Could you check a few things on this model? Use its own coordinates, in mm. Face numbers are marked on the shaded views. Give positions to 0.01 mm unless a question says otherwise; leave off trailing zeros. Order: outer loops, then holes, each group sorted by start corner. A loop starts at its lowest first (then second) coordinate and runs counter-clockwise, first axis right, second up. Notation, with made-up numbers: M 13,19.5 L 34,19.5 A31 ccw 34,43.5 Z; hole C 24,61 d6. An arc over 180 degrees is marked long. Use a Markdown table: item, result. Add a question column.
Item 1: Suppose I cut it at B-B on x = 10.5. Write out the boundary of the cut face in (y, z), plus the area to 3 significant figures.
Item 2: If I drill on L1, parallel to X at y = 14.75, z = -1; L2, parallel to Y at x = -20.5, z = 9; L3, parallel to Y at x = 17, z = 17, over which ranges is the centre line in solid material (lowest first)? Write a range as from..to.
Item 3: I'm going to push a flat-ended pin straight in: pin 1 Ø6 at (y, z) = (18, 7) entering from +X. Where does the tip first touch, or does it pass through?
Item 4: Suppose I cut it at C-C on x = 17. Write out the boundary of the cut face in (y, z), plus the area to 3 significant figures.
Item 5: Suppose I cut it at D-D on z = -5. Write out the boundary of the cut face in (x, y).
Item 6: If we mould it in two halves opening along Z, with no side actions, what happens to the marked faces 1, 2, 3 and 4? For each: released by +Z, released by -Z, zero draft, split by the parting line, or undercut.
Item 7: Suppose I cut it at A-A on y = 15. Write out the boundary of the cut face in (x, z), plus the area to 3 significant figures.
from build123d import *

# Parameters (mm, degrees)
SKETCH1_W               = 48
SKETCH1_H               = 45
BOSS_EXTRUDE1_DEPTH     = 30
SKETCH2_W               = 10.2
SKETCH2_H               = 20.2
CUT_EXTRUDE1_DEPTH      = 45
SKETCH3_R               = 4.15
CUT_EXTRUDE2_DEPTH      = 46
CUT_EXTRUDE3_DEPTH      = 1
CUT_EXTRUDE3_DEPTH_BACK = 31


with BuildPart() as part:
    # Sketch1 → Boss-Extrude1 (new body)
    with BuildSketch(Plane(origin=(0, 0, 0), x_dir=(1, 0, 0), z_dir=(0, 1, 0))):
        Rectangle(SKETCH1_W, SKETCH1_H)
    extrude(amount=BOSS_EXTRUDE1_DEPTH)

    # Sketch2 → Cut-Extrude1 (cut)
    with BuildSketch(Plane(origin=(24, 0, 0), x_dir=(0, 0, -1), z_dir=(1, 0, 0))):
        with Locations((-9, 15)):
            Rectangle(SKETCH2_W, SKETCH2_H)
    extrude(amount=-CUT_EXTRUDE1_DEPTH, mode=Mode.SUBTRACT)

    # Sketch3 → Cut-Extrude2 (cut, through all)
    with BuildSketch(Plane.XY.offset(22.5)):
        with Locations((-17, 15)):
            Circle(SKETCH3_R)
        with Locations((17, 15)):
            Circle(SKETCH3_R)
    extrude(amount=-CUT_EXTRUDE2_DEPTH, mode=Mode.SUBTRACT)

    # Sketch4 → Cut-Extrude3 (cut, two sides)
    with BuildSketch(Plane(origin=(0, 30, 0), x_dir=(1, 0, 0), z_dir=(0, 1, 0))) as cut_extrude3_sk:
        with BuildLine():
            Line((-7, 141.788608739), (-7, 22.5))
            ThreePointArc((-7, 22.5), (0, 15.5), (7, 22.5))
            Line((7, 22.5), (7, 141.788608739))
            Line((7, 141.788608739), (7, 380.365826216))
            Line((7, 380.365826216), (-7, 380.365826216))
            Line((-7, 380.365826216), (-7, 141.788608739))
        make_face()
    extrude(amount=CUT_EXTRUDE3_DEPTH, mode=Mode.SUBTRACT)
    extrude(cut_extrude3_sk.sketch, amount=-CUT_EXTRUDE3_DEPTH_BACK, mode=Mode.SUBTRACT)


solid = part.part
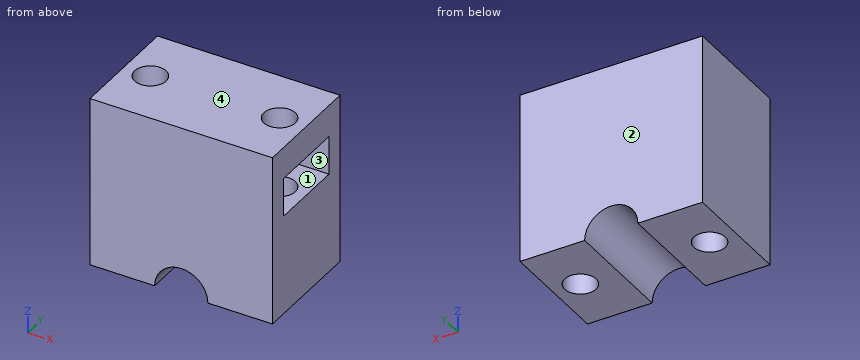
Findings below:
| question | item | result |
|---|---|---|
| 1 | outline | M 0,-22.5 L 30,-22.5 L 30,22.5 L 0,22.5 Z; hole M 4.9,3.9 L 25.1,3.9 L 25.1,14.1 L 4.9,14.1 Z |
| 1 | area | 1,140 mm^2 |
| 2 | L1 | x = -24..-21.14, -12.86..12.86, 21.14..24 |
| 2 | L2 | y = 0..4.9, 25.1..30 |
| 2 | L3 | y = 0..10.85, 19.15..30 |
| 3 | pin 1 | stops at x = -21 |
| 4 | outline | M 0,-22.5 L 10.85,-22.5 L 10.85,3.9 L 4.9,3.9 L 4.9,14.1 L 10.85,14.1 L 10.85,22.5 L 0,22.5 Z; M 19.15,-22.5 L 30,-22.5 L 30,22.5 L 19.15,22.5 L 19.15,14.1 L 25.1,14.1 L 25.1,3.9 L 19.15,3.9 Z |
| 4 | area | 855 mm^2 |
| 5 | outline | M -24,0 L 24,0 L 24,30 L -24,30 Z; hole C -17,15 d8.3; hole C 17,15 d8.3 |
| 6 | face 1 | undercut |
| 6 | face 2 | zero draft |
| 6 | face 3 | undercut |
| 6 | face 4 | released by +Z |
| 7 | outline | M -24,-22.5 L -21.15,-22.5 L -21.15,22.5 L -24,22.5 Z; M -12.85,-22.5 L -7,-22.5 A7 cw 7,-22.5 L 12.85,-22.5 L 12.85,3.9 L -12.85,3.9 Z; M -12.85,14.1 L 12.85,14.1 L 12.85,22.5 L -12.85,22.5 Z; M 21.15,-22.5 L 24,-22.5 L 24,3.9 L 21.15,3.9 Z; M 21.15,14.1 L 24,14.1 L 24,22.5 L 21.15,22.5 Z |
| 7 | area | 1,040 mm^2 |
